The drawing under review shows one solid part. Ordinate dimensions are in mm from its lowest x, y, z. A direction names the side the tool comes from. Coordinates: 2 decimals unless noted, no trailing zeros. Order: outer loops, then holes, each group sorted by start corner. A loop starts at its lowest first (then second) coordinate and runs counter-clockwise, first axis right, second up.
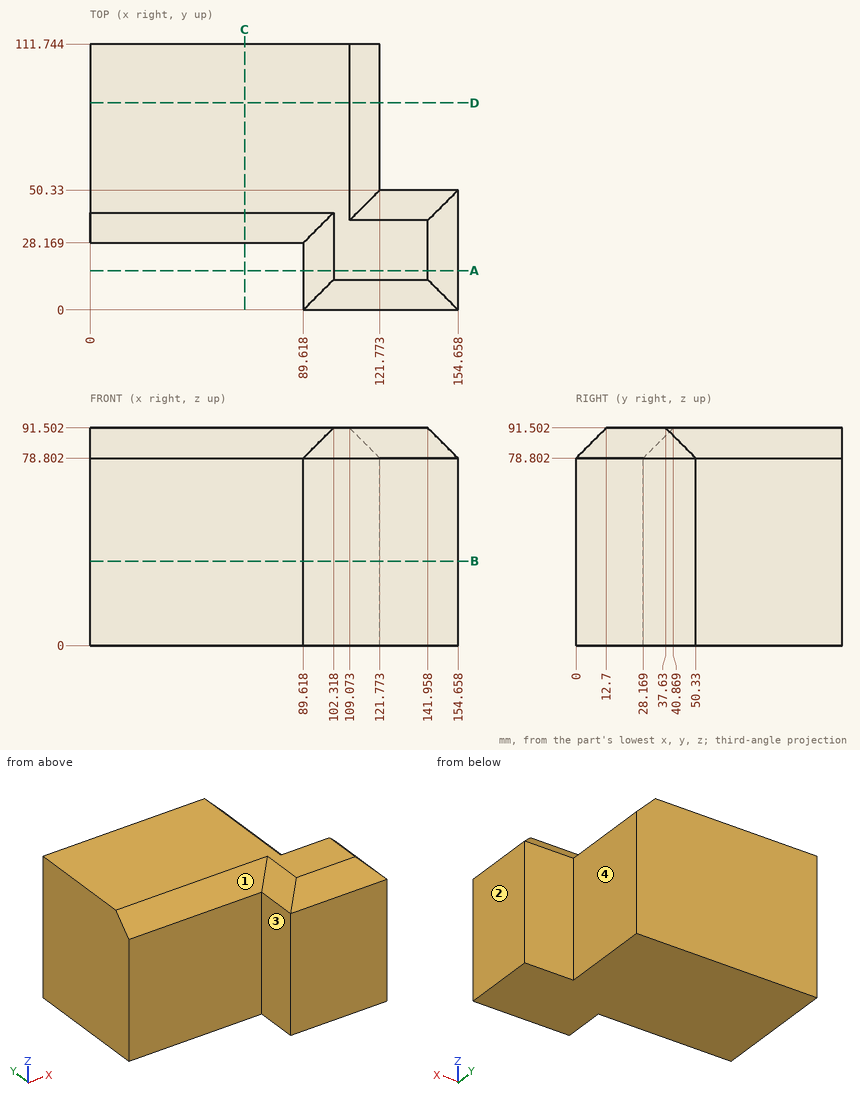
1. To check wall thickness, follow L1, parallel to X at y = 20, z = 57.5; L2, parallel to Y at x = 54.5, z = 23; L3, parallel to X at y = 57, z = 73.5. State the ranges of each line that lie inside material, in increasing order.
Answer below:
L1: x = 89.62 to 154.66
L2: y = 28.17 to 111.74
L3: x = 0 to 121.77
2. Take a section at D-D, the plane y = 87. Give the boundary of the cut face in (x, z), plus the area to 3 significant figures.
Answer below:
outline: (0, 0) - (121.77, 0) - (121.77, 78.8) - (109.07, 91.5) - (0, 91.5) - close
area: 11,100 mm2
3. Machinability: for the marked faces 1, 2, 3 and 4, which of the approach directions +Z, -Z, +X, -X, +Y, -Y give a long, thin tool a straight path to every point of the face, cutting with its end or side? Answer none if there is none.
Answer below:
face 1: +Z, -X, -Y
face 2: +Z, -Z, +X, +Y, -Y
face 3: +Z, -Z, -X, -Y
face 4: +Z, -Z, +X, +Y
4. Take a section at A-A, the plane y = 16.5. Give the boundary of the cut face in (x, z).
Answer below:
outline: (89.62, 0) - (154.66, 0) - (154.66, 78.8) - (141.96, 91.5) - (102.32, 91.5) - (89.62, 78.8) - close
5. Take a section at B-B, the plane z = 35.5. Give the boundary of the cut face in (x, y).
Answer below:
outline: (0, 28.17) - (89.62, 28.17) - (89.62, 0) - (154.66, 0) - (154.66, 50.33) - (121.77, 50.33) - (121.77, 111.74) - (0, 111.74) - close
6. Clearance check with flat-ended pins moving along their axes: pin 1 Ø8 at (x, z) = (31, 58.5) entering from -Y; pin 2 Ø5 at (y, z) = (17.5, 64) entering from -X; pin 3 Ø2 at (x, z) = (134, 19) entering from +Y. State where each tip first meets the part, or that it passes through.
Answer below:
pin 1: stops at y = 28.17
pin 2: stops at x = 89.62
pin 3: stops at y = 50.33
7. Take a section at C-C, the plane x = 65. Give the boundary of the cut face in (y, z), plus the area to 3 significant figures.
Answer below:
outline: (28.17, 0) - (111.74, 0) - (111.74, 91.5) - (40.87, 91.5) - (28.17, 78.8) - close
area: 7,570 mm2
